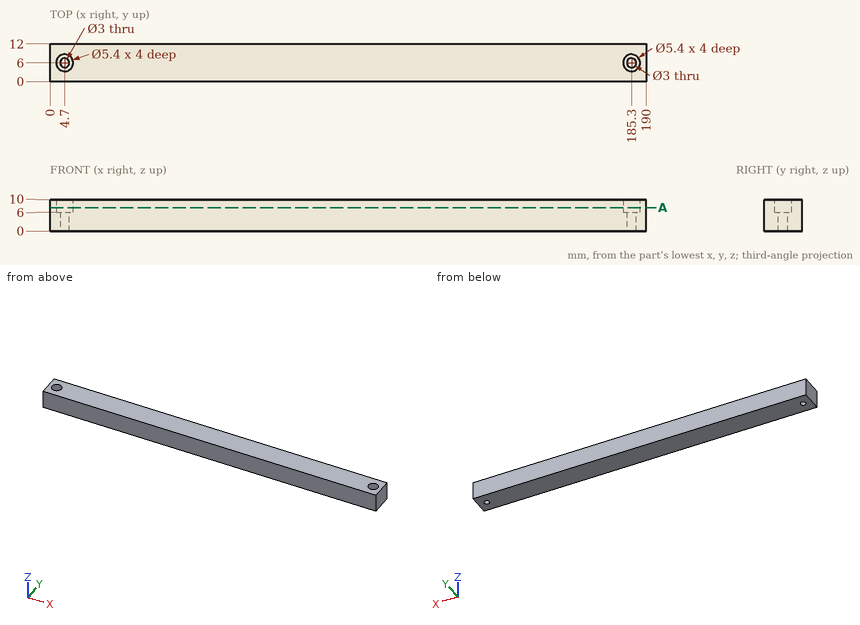
Here's the drawing with two shaded views (mm, measured from the low corner). I have some questions. Coordinates: 2 decimals unless noted, no trailing zeros. Order: outer loops, then holes, each group sorted by start corner. A loop starts at its lowest first (then second) coordinate and runs counter-clockwise, first axis right, second up.
Q1. Will these pins go through, and if not, where does the flat tip stop? pin 1 (6 mm diameter, centred on y = 5.5, z = 3, fed in from -X); pin 2 (4 mm diameter, centred on x = 185.3, y = 6, fed in from +Z); pin 3 (1.6 mm diameter, centred on x = 5, y = 6, fed in from +Z).
Q2. Suppose I cut it at A-A on z = 7.5. Please give me the cut outline in (x, y), and give its area (3 significant figures).
Q3. Please list where these lines run through material, in increasing order: L1, parallel to X at y = 6, z = 3.5; L2, parallel to X at y = 6, z = 8.7; L3, parallel to Y at x = 185.3, z = 8.75.
Answer:
1. pin 1: stops at x = 0
1. pin 2: stops at z = 6
1. pin 3: passes through
2. outline: (0, 0) - (190, 0) - (190, 12) - (0, 12) - close; hole circle Ø5.4 at (4.7, 6); hole circle Ø5.4 at (185.3, 6)
2. area: 2,230 mm2
3. L1: x = 0 to 3.2, 6.2 to 183.8, 186.8 to 190
3. L2: x = 0 to 2, 7.4 to 182.6, 188 to 190
3. L3: y = 0 to 3.3, 8.7 to 12
